The figure shows three views and two pictorial views of one solid part (mm, origin at its lowest corner). Answer the questions. A direction names the side the tool comes from. Round coordinates to 2 decimals unless told otherwise and drop trailing zeros. Order: outer loops, then holes, each group sorted by start corner. A loop starts at its lowest first (then second) coordinate and runs counter-clockwise, first axis right, second up. Notation, with made-up numbers: (18.25, 28) -> (36.25, 28) arc R32 ccw to (36.25, 65) -> close; hole circle Ø6 at (-33, 74.25). An arc over 180 degrees is marked (long way). One line per item, written item: value. Start each with the question number.
1. Section C-C (y = 42) is taken. Give the vertices of the cut face in (x, z), then the cut area to 3 significant figures.
2. Section D-D (y = 8) is taken. Give the vertices of the cut face in (x, z), then the cut area to 3 significant figures.
3. Flat-ended cylindrical pins translate along their axes: pin 1 Ø12 at (x, y) = (85, 21) entering from +Z; pin 2 Ø3 at (x, y) = (86, 33.5) entering from +Z; pin 3 Ø16.5 at (y, z) = (45, 40) entering from +X; pin 4 Ø2 at (x, y) = (41, 31) entering from -Z. Find the tip coordinate at first contact, or state that the pin passes through.
4. Consider line 1 (Y direction, x = 32.5, z = 32.5); line 2 (Z direction, x = 33.5, y = 12.5); line 3 (Y direction, x = 89.5, z = 12.5). Determine where each line is inside the solid, lowest interval first.
5. Section A-A (x = 52.5) is taken. Give the vertices of the cut face in (y, z), then the cut area to 3 significant figures.
6. Section B-B (y = 17) is taken. Give the vertices of the cut face in (x, z).
7. For the marked faces 1, 2 and 3, determine the directions among +Z, -Z, +X, -X, +Y, -Y from which every point of the face is accessible in a straight line to the end or side of a thin tool.
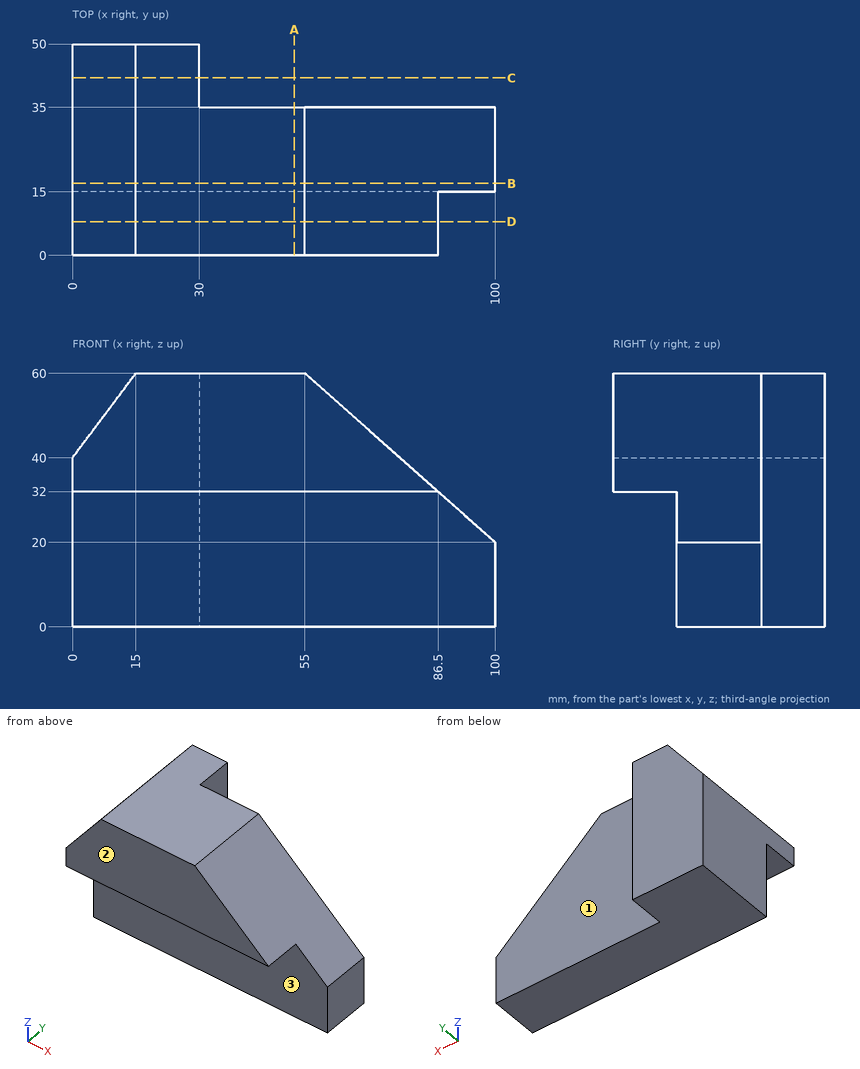
Answer:
1. outline: (0, 0) -> (30, 0) -> (30, 60) -> (15, 60) -> (0, 40) -> close
1. area: 1,650 mm^2
2. outline: (0, 32) -> (86.5, 32) -> (55, 60) -> (15, 60) -> (0, 40) -> close
2. area: 1,830 mm^2
3. pin 1: z = 38.67
3. pin 2: z = 33.78
3. pin 3: x = 30
3. pin 4: z = 0
4. line 1: 0 to 35
4. line 2: 32 to 60
4. line 3: 15 to 35
5. outline: (0, 32) -> (15, 32) -> (15, 0) -> (35, 0) -> (35, 60) -> (0, 60) -> close
5. area: 1,620 mm^2
6. outline: (0, 0) -> (100, 0) -> (100, 20) -> (55, 60) -> (15, 60) -> (0, 40) -> close
7. face 1: +Z, -Z, +X, +Y
7. face 2: +Z, -Z, +X, -X, -Y
7. face 3: -Z, +X, -X, -Y
